from build123d import *

# Parameters (mm, degrees)
F1_DEPTH = 12.5


with BuildPart() as f1:
    # F0 (on Front) → F1 (new body, symmetric)
    with BuildSketch(Plane.XZ):
        Polygon((-52.275904, -2.303776), (-56.58076, -4.034938), (-59.129985, -6.772994), (-59.483321, -11.718572), (-58.615414, -17.026151), (-53.908695, -23.969399), (-47.532922, -27.774831), (-39.488101, -29.844454), (-27.070367, -29.844454), (-15.620685, -27.374261), (-8.176722, -23.902636), (-2.902524, -17.126292), (-0.43233, -3.740512), (-1.700808, 0.432113), (-21.604338, 0.432113), (-42.484921, 3.422433), (-51.456425, 7.153944), (-60.507324, 14.140602), (-61.857025, 16.681206), (-61.857025, 19.777565), (-60.505413, 23.82762), (-58.821212, 25.652167), (-66.821156, 25.652167), (-69.010613, 19.168006), (-63.929948, 16.36101), (-64.350999, 12.655774), (-63.789598, 8.86633), (-61.936983, 6.143543), (-56.800178, 2.859358), (-45.349349, -1.669537), align=None)
        Polygon((-56.58076, -13.471695), (-56.58076, -8.311095), (-55.833608, -6.141283), (-53.763984, -4.288638), (-51.844578, -5.940998), (-48.100221, -7.287823), (-47.688644, -11.782673), (-45.15169, -16.889966), (-41.613301, -20.044469), (-37.056797, -21.262877), (-37.857941, -19.460302), (-39.994321, -18.325348), (-42.56466, -15.471273), (-43.516018, -11.799362), (-43.699614, -6.541855), (-40.31144, -1.70161), (-6.012463, -1.70161), (-4.259961, -3.621017), (-4.259961, -9.913336), (-5.311462, -15.905227), (-9.951422, -22.013951), (-16.243739, -24.667738), (-27.276158, -27.221385), (-39.276629, -27.388292), (-46.052973, -25.836074), (-52.32143, -22.025112), (-55.603315, -16.925327), align=None, mode=Mode.SUBTRACT)
    extrude(amount=F1_DEPTH, both=True)


solid = f1.part
CAD build for the part. Positions are in the model's coordinates, mm. A direction names the side the tool comes from. Coordinates: 2 decimals unless noted, no trailing zeros. Order: outer loops, then holes, each group sorted by start corner. A loop starts at its lowest first (then second) coordinate and runs counter-clockwise, first axis right, second up.
Item 1: Band-saw the part on A-A on x = -19. List the corners of the cut face in (y, z), plus the area to 3 significant figures.
Check sheet entries:
outline: (-12.5, -28.1) - (12.5, -28.1) - (12.5, -25.31) - (-12.5, -25.31) - close; (-12.5, -1.7) - (12.5, -1.7) - (12.5, 0.43) - (-12.5, 0.43) - close
area: 123 mm2
Item 2: Drill centre lines: L1, parallel to X at y = -7.75, z = -20; L2, parallel to Z at x = -51, y = 3.75; L3, parallel to X at y = 0.5, z = -24.5. Where is each one in solid material? Low to high.
Check sheet entries:
L1: x = -56.6 to -53.62, -41.66 to -37.62, -8.42 to -5.14
L2: z = -25.71 to -22.83, -6.24 to -2.19, 0.57 to 6.96
L3: x = -53.02 to -48.25, -15.85 to -9.46
Item 3: Pin check, flat tips, straight feed: pin 1 Ø4 at (x, y) = (-41, 0) entering from +Z; pin 2 Ø1.5 at (y, z) = (-5, 18.5) entering from +X; pin 3 Ø5.5 at (y, z) = (3, -11) entering from +X. Stop position of each tip, or through.
Check sheet entries:
pin 1: stops at z = 3.64
pin 2: stops at x = -61.86
pin 3: stops at x = -1.26
Item 4: Two-plate mould, pull along X, no slides. Class faces 1 (the face through (-54.4, -0.18, -3.16)), 2 (the face through (-54.813, -0.175, -5.228)), 3 (the face through (-46.908, -0.175, 5.262)): +X half, -X half, draft (parallel to the pull), parting line (faces both ways), or undercut.
Check sheet entries:
face 1: -X half
face 2: undercut
face 3: +X half
Item 5: 3-axis set-ups, long thin cutter, end or side, ignore diameter. For faces 4 (the face through (-12, 0, 0.432)), 5 (the face through (-59.4, -0.18, 4.52)), 6 (the face through (-7.6, -0.18, -18.92)), 7 (the face through (-61.857, 0, 18)): which of +Z, -Z, +X, -X, +Y, -Y reach the whole face in a straight line?
Check sheet entries:
face 4: +Z, +X, +Y, -Y
face 5: -X, +Y, -Y
face 6: +Y, -Y
face 7: +X, +Y, -Y
